Study the drawing (mm; zero at the part's minimum x, y, z) and answer. A direction names the side the tool comes from. Give positions to 0.01 mm unless a question says otherwise; leave off trailing zeros. Loops run counter-clockwise (first coordinate to the right, second up) from the corner with the lowest first, then second, coordinate; pieces in that order, holes last. Notation, with made-up numbers: (-7.5, 57.25) - (6.5, 57.25) arc R20 ccw to (6.5, 75.25) - close; hole circle Ø8 at (16, -17.75). An arc over 180 degrees is marked (long way). Write item = value, one per line. Start each with the question number.
1) The mould has two halves that part along Y. Classify the marked faces 1, 2 and 3: +Y half, -Y half, draft (parallel to the pull), parting line (faces both ways), or undercut.
2) Which of the six approach directions +Z, -Z, +X, -X, +Y, -Y give full straight-line access (tool end or side, diameter ignored) to the marked faces 4 and 5?
3) The part is cut by section B-B on z = 7.5. Write down the section's boundary in (x, y).
4) The part is cut by section A-A on x = 0.75. Write down the section's boundary in (y, z), plus the area to 3 significant figures.
5) Consider probe 1 along Y at (x, z) = (4.5, 7.25); probe 2 along Z at (x, y) = (2.5, 26.5); probe 3 along X at (y, z) = (16, 8.75). Determine where each line is inside the solid, lowest interval first.
6) The part is cut by section C-C on y = 26.5. Write down the section's boundary in (x, z).
7) The part is cut by section D-D on x = 5. Write down the section's boundary in (y, z), plus the area to 3 significant figures.
8) Flat-ended cylindrical pins translate along their axes: P1, Ø2.5, axis at y = 26.5, z = 7.5, coming from the +X side; P2, Ø1.5, axis at x = 2, z = 5, coming from the +Y side; P3, Ø1, axis at x = 2, z = 5, coming from the +Y side; P4, Ø2.5, axis at y = 5, z = 7.5, coming from the -X side. Find the tip coordinate at first contact, or state that the pin passes through.
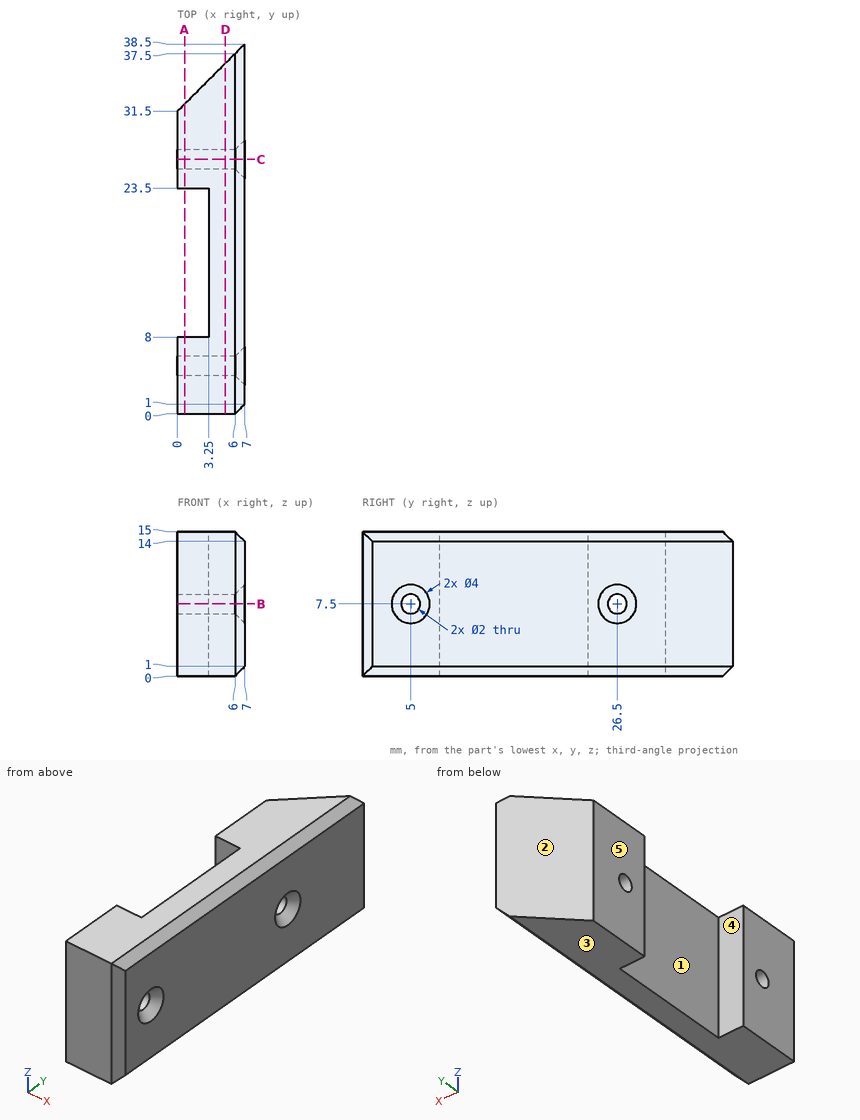
Answer below:
q1.face_1 = undercut
q1.face_2 = +Y half
q1.face_3 = draft
q2.face_4 = +Z, -Z, -X
q2.face_5 = +Z, -Z, -X, +Y, -Y
q3.outline = (0, 0) - (6, 0) - (7, 1) - (7, 3) - (6, 4) - (0, 4) - close; (0, 6) - (6, 6) - (7, 7) - (7, 24.5) - (6, 25.5) - (0, 25.5) - (0, 23.5) - (3.25, 23.5) - (3.25, 8) - (0, 8) - close; (0, 27.5) - (6, 27.5) - (7, 28.5) - (7, 38.5) - (0, 31.5) - close
q4.outline = (0, 0) - (8, 0) - (8, 15) - (0, 15) - close; (23.5, 0) - (32.25, 0) - (32.25, 15) - (23.5, 15) - close; hole circle Ø2 at (5, 7.5); hole circle Ø2 at (26.5, 7.5)
q4.area = 245 mm2
q5.probe_1 = 0 to 4.03, 5.97 to 25.53, 27.47 to 36
q5.probe_2 = 0 to 6.5, 8.5 to 15
q5.probe_3 = 3.25 to 7
q6.outline = (0, 0) - (6, 0) - (7, 1) - (7, 5.5) - (6, 6.5) - (0, 6.5) - close; (0, 8.5) - (6, 8.5) - (7, 9.5) - (7, 14) - (6, 15) - (0, 15) - close
q7.outline = (0, 0) - (36.5, 0) - (36.5, 15) - (0, 15) - close; hole circle Ø2 at (5, 7.5); hole circle Ø2 at (26.5, 7.5)
q7.area = 541 mm2
q8.P1 = 6.25
q8.P2 = 34.25
q8.P3 = 34
q8.P4 = 0
